from build123d import *

# Parameters (mm, degrees)
BOSS_EXTRUDE1_REACH     = 57.084
SENSOR_R                = 6.35
SKETCH4_R               = 4.445
CUT_EXTRUDE1_DEPTH      = 2.54
CUT_EXTRUDE2_REACH      = 57.084
CUT_EXTRUDE2_END_RADIUS = 7.9375


with BuildPart() as part:
    # Sketch1 → mainBody (revolve)
    with BuildSketch(Plane(origin=(0, 0, 0), x_dir=(0, 0, -1), z_dir=(1, 0, 0)), mode=Mode.PRIVATE) as mainbody_sk:
        Polygon((-9.525, 0), (-7.9375, 0), (-7.9375, -30.492216058), (0, -30.492216058), (0, -50.8), (-9.525, -34.302216058), align=None)
    revolve(mainbody_sk.sketch.rotate(Axis((0, 0, 0), (0, 1, 0)), 180), axis=Axis((0, 0, 0), (0, 1, 0)))

    # sensor → Boss-Extrude1 (add, up to next)
    with BuildSketch(Plane(origin=(9.525, 0, 0), x_dir=(0, 0, -1), z_dir=(1, 0, 0)), mode=Mode.PRIVATE) as boss_extrude1_sk1:
        with Locations((0, -25.412216058)):
            Circle(SENSOR_R)
    boss_extrude1_tool1 = extrude(boss_extrude1_sk1.sketch, amount=-BOSS_EXTRUDE1_REACH, mode=Mode.PRIVATE) - part.part
    add(boss_extrude1_tool1.solids().sort_by_distance((9.525, -25.412216, 0))[0])
    add(boss_extrude1_tool1.solids().sort_by_distance((9.525, -25.412216, 0))[1])

    # Sketch4 → Cut-Extrude1 (cut)
    with BuildSketch(Plane(origin=(9.525, 0, 0), x_dir=(0, 0, -1), z_dir=(1, 0, 0))):
        with Locations((0, -25.412216058)):
            Circle(SKETCH4_R)
    extrude(amount=-CUT_EXTRUDE1_DEPTH, mode=Mode.SUBTRACT)

    # Cut-Extrude2: up to this cylinder (the profile starts outside it)
    cut_extrude2_end = Plane(origin=(0, -14.917784, 0), z_dir=(0, -1, 0)) * Cylinder(CUT_EXTRUDE2_END_RADIUS, 131.043, mode=Mode.PRIVATE)
    # Sketch5 → Cut-Extrude2 (cut, up to the surface)
    with BuildSketch(Plane(origin=(9.525, 0, 0), x_dir=(0, 0, -1), z_dir=(1, 0, 0)), mode=Mode.PRIVATE) as cut_extrude2_sk1:
        with BuildLine():
            Line((-1.5875, -7.886216058), (1.5875, -7.886216058))
            Line((1.5875, -7.886216058), (1.5875, -20.132735353))
            ThreePointArc((1.5875, -20.132735353), (0, -22.237216058), (-1.5875, -20.132735353))
            Line((-1.5875, -20.132735353), (-1.5875, -7.886216058))
        make_face()
    cut_extrude2_tool1 = extrude(cut_extrude2_sk1.sketch, amount=-CUT_EXTRUDE2_REACH, mode=Mode.PRIVATE) - cut_extrude2_end
    add(cut_extrude2_tool1.solids().sort_by_distance((9.525, -14.917784, 0))[0], mode=Mode.SUBTRACT)


solid = part.part
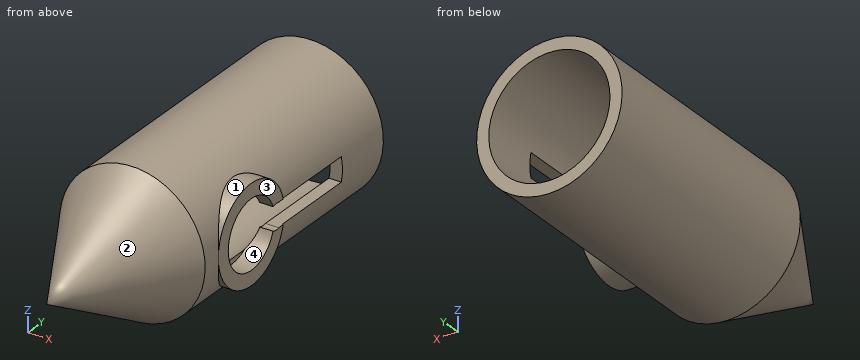
Work out the finished part from the listing and answer in its coordinate system (mm). Face numbers are marked on the shaded views. Give positions to 0.01 mm unless a question says otherwise; leave off trailing zeros. Order: outer loops, then holes, each group sorted by start corner. A loop starts at its lowest first (then second) coordinate and runs counter-clockwise, first axis right, second up. Notation, with made-up numbers: (78, 1.25) -> (111, 1.25) arc R15 ccw to (111, 9.25) -> close; hole circle Ø3 at (20.25, -12.75). An arc over 180 degrees is marked (long way). Answer as a JSON object with one key per item and string values. Group by question number.
1. Section C-C on y = -38 is taken. Determine the outline of the cut face in (x, z).
2. Consider line 1 along Z through (x, y) = (8.75, -33.5); line 2 along X through (y, z) = (-25.5, 0) (1 decimal); line 3 along Z through (x, y) = (3.5, -21.5). Determine where each line is inside the solid, lowest interval first. Write a range as [from, to].
3. The mould has two halves that part along Y. Classify the marked faces 1, 2, 3 and 4: released by +Y, released by -Y, zero draft, split by the parting line, or undercut.
4. Flat-ended cylindrical pins translate along their axes: pin 1 Ø1 at (x, y) = (-0.5, -34.5) entering from -Z; pin 2 Ø0.5 at (y, z) = (-26.5, 4) entering from +X (3 decimals); pin 3 Ø5 at (x, z) = (-1.5, -4.5) entering from +Y; pin 4 Ø1.4 at (x, z) = (8.5, -1) entering from -Y. Find the tip coordinate at first contact, or state that the pin passes through.
Result sheet:
{
 "1": {"outline": "circle Ø14.78 at (0, 0)"},
 "2": {"line 1": "z = [-3.76, 3.76]", "line 2": "x = [-9.5, -7.9]", "line 3": "z = [-8.86, -7.12], [7.12, 8.86]"},
 "3": {"face 1": "split by the parting line", "face 2": "released by -Y", "face 3": "zero draft", "face 4": "undercut"},
 "4": {"pin 1": "stops at z = -9.52", "pin 2": "stops at x = 6.985", "pin 3": "stops at y = -30.49", "pin 4": "stops at y = -37.19"}
}
